from build123d import *

# Parameters (mm, degrees)
ESQUISSE1_W        = 70
ESQUISSE1_H        = 70
BOSS_EXTRU_1_DEPTH = 2
ESQUISSE3_W        = 14.4
ESQUISSE3_H        = 8.4
ESQUISSE3_W_2      = 10.4
ESQUISSE3_H_2      = 4.4
BOSS_EXTRU_3_DEPTH = 15
D_POUILLE3_ANGLE   = 2
CONG_1_R           = 2


with BuildPart() as part:
    # Esquisse1 → Boss.-Extru.1 (new body)
    with BuildSketch(Plane.XY):
        Rectangle(ESQUISSE1_W, ESQUISSE1_H)
    extrude(amount=BOSS_EXTRU_1_DEPTH)

    # Esquisse3 → Boss.-Extru.3 (add)
    with BuildSketch(Plane.XZ.offset(35)):
        with Locations((0, -2.3)):
            Rectangle(ESQUISSE3_W, ESQUISSE3_H)
        with Locations((0, -2.3)):
            Rectangle(ESQUISSE3_W_2, ESQUISSE3_H_2, mode=Mode.SUBTRACT)
    extrude(amount=-BOSS_EXTRU_3_DEPTH)

    # Dépouille3
    d_pouille3_faces = [part.faces().sort_by_distance(p)[0] for p in [
        (0, -27.5, -0.1),
        (-5.2, -27.5, -2.3),
        (0, -27.5, -4.5),
        (5.2, -27.5, -2.3),
    ]]
    draft(d_pouille3_faces, Plane(origin=(-35, -35, 2), x_dir=(0, 0, -1), z_dir=(0, -1, 0)), D_POUILLE3_ANGLE)

    # Congé1
    cong_1_edges = [part.edges().sort_by_distance(p)[0] for p in [
        (35, -35, 1),
        (-35, -35, 1),
        (-35, 35, 1),
        (35, 35, 1),
    ]]
    fillet(cong_1_edges, radius=CONG_1_R)


solid = part.part
The listing builds one solid part. Answer for the finished solid, in the listing's coordinates (mm). A direction names the side the tool comes from. Coordinates: 2 decimals unless noted, no trailing zeros. Loops run counter-clockwise (first coordinate to the right, second up) from the corner with the lowest first, then second, coordinate; pieces in that order, holes last. Notation, with made-up numbers: M 48,0 L 54,0 A28 ccw 54,38 Z; hole C -26,18 d10. An arc over 180 degrees is marked long. Answer in a Markdown table with one row per item.
1) Find section A-A (z = -2.25). Determine the outline of the cut face in (x, y).
Answers below:
| item | result |
|---|---|
| outline | M -7.2,-35 L -5.2,-35 L -4.68,-20 L -7.2,-20 Z; M 4.68,-20 L 5.2,-35 L 7.2,-35 L 7.2,-20 Z |
2) Find section D-D (y = 0.5). Determine the outline of the cut face in (x, z).
Answers below:
| item | result |
|---|---|
| outline | M -35,0 L 35,0 L 35,2 L -35,2 Z |
3) Find the intervals of material crossed by probe 1 along Z at (x, y) = (7.5, -7.5); probe 2 along Y at (x, z) = (2, -5.25); probe 3 along X at (y, z) = (-22.5, -5.75), in increasing order.
Answers below:
| item | result |
|---|---|
| probe 1 | 0 to 2 |
| probe 2 | -35 to -20 |
| probe 3 | -7.2 to 7.2 |
4) Find section B-B (x = -1). Determine the outline of the cut face in (y, z), then the cut area to 3 significant figures.
Answers below:
| item | result |
|---|---|
| outline | M -35,-6.5 L -20,-6.5 L -20,-3.98 L -35,-4.5 Z; M -35,-0.1 L -20,-0.62 L -20,0 L 35,0 L 35,2 L -35,2 Z |
| area | 179 mm^2 |
5) Given pin 1 (2 mm diameter, centred on y = -30.5, z = -4, fed in from -X); pin 2 (2 mm diameter, centred on y = -6.5, z = -2.5, fed in from -X); pin 3 (10 mm diameter, centred on x = 27.5, y = -5.5, fed in from -Z); pin 4 (3 mm diameter, centred on y = -29.5, z = -2, fed in from +X), each flat-ended and moving along its own axis, determine where each tip first touches the part or whether it passes through.
Answers below:
| item | result |
|---|---|
| pin 1 | x = -7.2 |
| pin 2 | through |
| pin 3 | z = 0 |
| pin 4 | x = 7.2 |
6) Which of the six approach directions +Z, -Z, +X, -X, +Y, -Y give full straight-line access (tool end or side, diameter ignored) to faces 1 (the flat face through (-7.2, -28, -3)), 2 (the flat face through (7.2, -28, -3)), 3 (the flat face through (0, -20, -5)), 4 (the flat face through (-35, 0, 1))?
Answers below:
| item | result |
|---|---|
| face 1 | -Z, -X, +Y, -Y |
| face 2 | -Z, +X, +Y, -Y |
| face 3 | -Z, +X, -X, +Y |
| face 4 | +Z, -Z, -X, +Y, -Y |
7) Find section C-C (y = -30). Determine the outline of the cut face in (x, z).
Answers below:
| item | result |
|---|---|
| outline | M -35,0 L -7.2,0 L -7.2,-6.5 L 7.2,-6.5 L 7.2,0 L 35,0 L 35,2 L -35,2 Z; hole M -5.03,-4.33 L 5.03,-4.33 L 5.03,-0.27 L -5.03,-0.27 Z |
8) Determine the mould class of faces 5 (the flat face through (0, 0, 2)), 6 (the cylindrical face through (34.4, 34.43, 1.01)), 7 (the flat face through (0, -28, -6.5)) for opening direction Z: released by +Z, released by -Z, zero draft, split by the parting line, or undercut.
Answers below:
| item | result |
|---|---|
| face 5 | released by +Z |
| face 6 | zero draft |
| face 7 | released by -Z |
